```python
from build123d import *

# Parameters (mm, degrees)
CIRCLE004_R      = 2
EXTRUDE090_DEPTH = 5
CIRCLE006_R      = 2
EXTRUDE091_DEPTH = 5
RECTANGLE063_W   = 6
RECTANGLE063_H   = 6
EXTRUDE077_DEPTH = 7.5
RECTANGLE003_W   = 17
RECTANGLE003_H   = 60
EXTRUDE002_DEPTH = 5


with BuildPart() as extrude090:
    # Circle004 → Extrude090 (new body)
    with BuildSketch(Plane(origin=(-140, 10, 55), x_dir=(0, -1, 0), z_dir=(-1, 0, 0))):
        Circle(CIRCLE004_R)
    extrude(amount=-EXTRUDE090_DEPTH)


with BuildPart() as extrude091:
    # Circle006 → Extrude091 (new body)
    with BuildSketch(Plane(origin=(-140, 10, 25), x_dir=(0, -1, 0), z_dir=(-1, 0, 0))):
        Circle(CIRCLE006_R)
    extrude(amount=-EXTRUDE091_DEPTH)


with BuildPart() as extrude077:
    # Rectangle063 → Extrude077 (new body)
    with BuildSketch(Plane(origin=(-250, 6, 64), x_dir=(0, -1, 0), z_dir=(-1, 0, 0))):
        with Locations((3, 3)):
            Rectangle(RECTANGLE063_W, RECTANGLE063_H)
    extrude(amount=-EXTRUDE077_DEPTH)


with BuildPart() as extrude077_1:
    # Extrude077 placement: moved
    add(extrude077.part.moved(Location((110, 0, 0))))


with BuildPart() as cut009:
    # Rectangle003 → Extrude002 (new body)
    with BuildSketch(Plane(origin=(0, 0, 10), x_dir=(0, 1, 0), z_dir=(1, 0, 0))):
        with Locations((8.5, 30)):
            Rectangle(RECTANGLE003_W, RECTANGLE003_H)
    extrude(amount=EXTRUDE002_DEPTH)


with BuildPart() as cut009_1:
    # Extrude002 placement: moved
    add(cut009.part.moved(Location((-140, 0, 0))))

    # Cut: cut Extrude077
    add(extrude077_1.part, mode=Mode.SUBTRACT)

    # Cut008: cut Extrude091
    add(extrude091.part, mode=Mode.SUBTRACT)

    # Cut009: cut Extrude090
    add(extrude090.part, mode=Mode.SUBTRACT)


with BuildPart() as cut009_2:
    # Cut009 placement: moved
    add(cut009_1.part.moved(Location((-2.5, 0, 0))))


solid = cut009_2.part
```
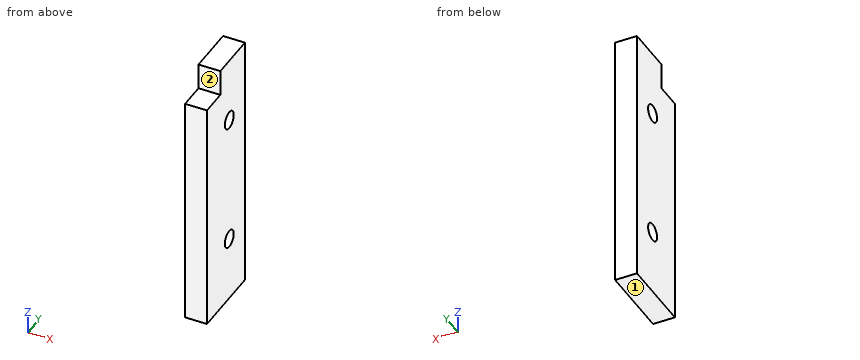
For this review, take the finished solid that the model builds, in its own axes (mm). Face numbers are marked on the shaded views. A direction names the side the tool comes from. Coordinates: 2 decimals unless noted, no trailing zeros. Order: outer loops, then holes, each group sorted by start corner. A loop starts at its lowest first (then second) coordinate and runs counter-clockwise, first axis right, second up. Notation, with made-up numbers: (-21.75, 23) -> (13.25, 23) arc R13 ccw to (13.25, 43) -> close; hole circle Ø3 at (-13, 67). An arc over 180 degrees is marked (long way). Answer as CSV lines item,"result".
Q1. We need section A-A (z = 25). State the section outline as (x, y) points.
Model answer:
outline,"(-142.5, 0) -> (-137.5, 0) -> (-137.5, 8) -> (-142.5, 8) -> close; (-142.5, 12) -> (-137.5, 12) -> (-137.5, 17) -> (-142.5, 17) -> close"
Q2. Wall thickness on line 1 along Z through (x, y) = (-139.5, 10); line 2 along Z through (x, y) = (-139.3, 11.5); line 3 along Z through (x, y) = (-142.15, 3.5): over which ranges is each line inside the solid? List them lowest first. Write a range as [from, to].
Model answer:
line 1,"z = [10, 23], [27, 53], [57, 70]"
line 2,"z = [10, 23.68], [26.32, 53.68], [56.32, 70]"
line 3,"z = [10, 64]"
Q3. We need section B-B (y = 10). State the section outline as (x, z) points, plus the area to 3 significant figures.
Model answer:
outline,"(-142.5, 10) -> (-137.5, 10) -> (-137.5, 23) -> (-142.5, 23) -> close; (-142.5, 27) -> (-137.5, 27) -> (-137.5, 53) -> (-142.5, 53) -> close; (-142.5, 57) -> (-137.5, 57) -> (-137.5, 70) -> (-142.5, 70) -> close"
area,"260 mm2"
Q4. For the marked faces 1 and 2, list the 3-axis set-ups (+Z, -Z, +X, -X, +Y, -Y) from which the entire face can be reached by the end or side of a thin tool; tool diameter is ignored.
Model answer:
face 1,"-Z, +X, -X, +Y, -Y"
face 2,"+Z, +X, -X, -Y"
Q5. We need section C-C (x = -139.75). State the section outline as (y, z) points, plus the area to 3 significant figures.
Model answer:
outline,"(0, 10) -> (17, 10) -> (17, 70) -> (6, 70) -> (6, 64) -> (0, 64) -> close; hole circle Ø4 at (10, 25); hole circle Ø4 at (10, 55)"
area,"959 mm2"
Q6. We need section D-D (y = 4.5). State the section outline as (x, z) points, plus the area to 3 significant figures.
Model answer:
outline,"(-142.5, 10) -> (-137.5, 10) -> (-137.5, 64) -> (-142.5, 64) -> close"
area,"270 mm2"
Q7. Clearance check with flat-ended pins moving along their axes: pin 1 Ø4.5 at (y, z) = (10, 25) entering from -X; pin 2 Ø1 at (x, y) = (-139, 4) entering from +Z. State where each tip first meets the part, or that it passes through.
Model answer:
pin 1,"stops at x = -142.5"
pin 2,"stops at z = 64"
